Geometry: final body of the model. Coordinates: model frame, mm. A direction names the side the tool comes from. Give positions to 0.01 mm unless a question says otherwise; leave off trailing zeros. Write each loop counter-clockwise with the first axis right and the second up, starting at its lowest first coordinate (ties: lowest second). Pieces come first, ordered by that corner, then holes.
Q1. Line query: L1, parallel to Z at x = 65.75, y = 4.75; L2, parallel to Y at x = 52.25, z = 34.5; L3, parallel to Z at x = 67.5, y = 3.25. Output: solid intervals per line, ascending.
Q2. Pin query (flat end, axial travel): pin 1 (6.5 mm diameter, centred on x = 48, z = 41, fed in from -Y). Return the tip coordinate at first contact, or that it passes through.
Q3. Cut plane C-C on x = 46.5. Return the cut outline in (y, z).
Q4. Draft query along X for faces 1 (the face through (51, 0, 37)), 2 (the face through (39.93, 2.46, 43.97)), 3 (the face through (63, 2, 45.925)), 4 (the face through (68.93, 7, 37)). Return one class per face: pulls with the +X half, pulls with the -X half, needs draft (parallel to the pull), parting line crosses it, or undercut.
Q5. Cut plane A-A on y = 3. Return the cut outline in (x, z), plus the area to 3 significant figures.
Q6. Cut plane B-B on z = 32.5. Return the cut outline in (x, y), plus the area to 3 significant figures.
Q7. Cut plane D-D on x = 55. Return the cut outline in (y, z), plus the area to 3 significant figures.
Q8. Reachability of faces 5 (the face through (38.93, 7, 37)), 6 (the face through (63, 2, 41.925)) from +Z, -Z, +X, -X, +Y, -Y: full face, straight path, thin tool, end or side. Return the list, or none.
Solid Edge part; units mm, degrees
sketch "Sketch1" plane through (0, 0, 0) normal (0, -1, 0) x (1, 0, 0)
  line L0 (38.9305, 51.9251) -> (68.9305, 51.9251)
  line L1 (68.9305, 51.9251) -> (68.9305, 21.9251)
  line L2 (68.9305, 21.9251) -> (38.9305, 21.9251)
  line L3 (38.9305, 21.9251) -> (38.9305, 51.9251)
  dimension "D1" = 38.9305
  dimension "D2" = 68.9305
extrude "Protrusion1" add sketch "Sketch1" against normal blind 15
sketch "Sketch2" plane through (63.9305, 0, 41.9251) normal (0, -1, 0) x (1, 0, 0)
  line L0 (-8, -5) -> (-8, -10)
  arc A0 (-8, -10) -> (-12, -10) centre (-10, -10) cw
  line L1 (-12, -10) -> (-12, -5)
  arc A1 (-12, -5) -> (-17, 0) centre (-17, -5) ccw
  line L2 (-17, 0) -> (-22, 0)
  arc A2 (-22, 0) -> (-22, 4) centre (-22, 2) cw
  line L3 (-22, 4) -> (-17, 4)
  arc A3 (-17, 4) -> (-14, 7) centre (-17, 7) ccw
  arc A4 (-14, 7) -> (-6, 7) centre (-10, 4) cw
  arc A5 (-3, 4) -> (-6, 7) centre (-3, 7) cw
  line L4 (2, 4) -> (-3, 4)
  arc A6 (2, 0) -> (2, 4) centre (2, 2) ccw
  line L5 (-3, 0) -> (2, 0)
  arc A7 (-8, -5) -> (-3, 0) centre (-3, -5) cw
  dimension "D1" = 8
  dimension "D2" = 12
  dimension "D3" = 3
  dimension "D4" = 17
  dimension "D5" = 22
  dimension "D6" = 2
extrude "ExtrudedCutout_4" cut sketch "Sketch2" against normal blind 5
sketch "Sketch3" plane through (63.9305, 5, 35.4251) normal (0, -1, 0) x (1, 0, 0)
  circle A0 centre (-10, 10) radius 2.5
  dimension "D1" = 10
extrude "ExtrudedProtrusion_3" add sketch "Sketch3" along normal blind 5
Data:
1. L1: z = 21.93 to 41.93, 45.93 to 51.93
1. L2: y = 5 to 15
1. L3: z = 21.93 to 42.69, 45.16 to 51.93
2. pin 1: stops at y = 0
3. outline: (0, 21.93) - (15, 21.93) - (15, 51.93) - (0, 51.93) - (0, 45.93) - (5, 45.93) - (5, 41.93) - (0, 41.93) - close
4. face 1: needs draft
4. face 2: undercut
4. face 3: undercut
4. face 4: pulls with the +X half
5. outline: (38.93, 21.93) - (68.93, 21.93) - (68.93, 51.93) - (38.93, 51.93) - close; circle Ø5 at (53.93, 45.43); hole (41.93, 41.93) - (46.93, 41.93) arc R5 cw to (51.93, 36.93) - (51.93, 31.93) arc R2 ccw to (55.93, 31.93) - (55.93, 36.93) arc R5 cw to (60.93, 41.93) - (65.93, 41.93) arc R2 ccw to (65.93, 45.93) - (60.93, 45.93) arc R3 cw to (57.93, 48.93) arc R5 ccw to (49.93, 48.93) arc R3 cw to (46.93, 45.93) - (41.93, 45.93) arc R2 ccw to start
5. area: 715 mm2
6. outline: (38.93, 0) - (51.93, 0) - (51.93, 5) - (55.93, 5) - (55.93, 0) - (68.93, 0) - (68.93, 15) - (38.93, 15) - close
6. area: 430 mm2
7. outline: (0, 21.93) - (15, 21.93) - (15, 51.93) - (0, 51.93) - (0, 50.81) - (5, 50.81) - (5, 47.68) - (0, 47.68) - (0, 43.17) - (5, 43.17) - (5, 30.24) - (0, 30.24) - close
7. area: 370 mm2
8. face 5: +Z, -Z, -X, +Y, -Y
8. face 6: -Y
